Read the model definition and answer for the solid it produces. Units are mm, in the model's axes. A direction names the side the tool comes from. Give positions to 0.01 mm unless a question says otherwise; leave off trailing zeros. Write each loop counter-clockwise with the first axis right and the second up, starting at its lowest first coordinate (ties: lowest second). Pieces come first, ordered by that corner, then holes. Notation, with made-up numbers: M 45.5,-30 L 98.5,-30 A32 cw 98.5,3 Z; hole C 59.25,-16.75 d11. An arc over 180 degrees is marked long. Put each result on its own line as item: value.
from build123d import *

# Parameters (mm, degrees)
SKETCH_1_R               = 18.5
EXTRUDE_1_DEPTH          = 21.5
SKETCH_2_R               = 6
EXTRUDE_2_DEPTH          = 6
SKETCH_3_R               = 3
EXTRUDE_3_DEPTH          = 15
CUT_EXTRUDE_1_DEPTH      = 1
CUT_EXTRUDE_1_DEPTH_BACK = 11.5
SKETCH_5_R               = 1.5
CUT_EXTRUDE_2_DEPTH      = 5
SKETCH_6_R               = 16.4
EXTRUDE_4_DEPTH          = 22
SKETCH_7_R               = 1
EXTRUDE_5_DEPTH          = 6.84
SKETCH_8_R               = 3.75
EXTRUDE_6_DEPTH          = 3.5
SKETCH_9_W               = 0.5
SKETCH_9_H               = 3
EXTRUDE_7_DEPTH          = 6.64


with BuildPart() as part:
    # 草图1 → 凸台-拉伸1 (new body)
    with BuildSketch(Plane.XY):
        Circle(SKETCH_1_R)
    extrude(amount=EXTRUDE_1_DEPTH)

    # 草图2 → 凸台-拉伸2 (add)
    with BuildSketch(Plane(origin=(0, 0, 0), x_dir=(-1, 0, 0), z_dir=(0, 0, -1))):
        with Locations((0, 7)):
            Circle(SKETCH_2_R)
    extrude(amount=EXTRUDE_2_DEPTH)

    # 草图3 → 凸台-拉伸3 (add)
    with BuildSketch(Plane(origin=(0, 0, -6), x_dir=(-1, 0, 0), z_dir=(0, 0, -1))):
        with Locations((0, 7)):
            Circle(SKETCH_3_R)
    extrude(amount=EXTRUDE_3_DEPTH)

    # 草图4 → 切除-拉伸1 (cut, two sides)
    with BuildSketch(Plane(origin=(0, 0, -21), x_dir=(-1, 0, 0), z_dir=(0, 0, -1))) as cut_extrude_1_sk:
        Polygon((-80.661429966, 9.5), (-1.658312395, 9.5), (1.658312395, 9.5), (80.661429966, 9.5), (80.661429966, 167.506235142), (-80.661429966, 167.506235142), align=None)
    extrude(amount=CUT_EXTRUDE_1_DEPTH, mode=Mode.SUBTRACT)
    extrude(cut_extrude_1_sk.sketch, amount=-CUT_EXTRUDE_1_DEPTH_BACK, mode=Mode.SUBTRACT)

    # 草图5 → 切除-拉伸2 (cut)
    with BuildSketch(Plane(origin=(0, 0, 0), x_dir=(-1, 0, 0), z_dir=(0, 0, -1))):
        with Locations((15.5, 0)):
            Circle(SKETCH_5_R)
        with Locations((7.75, -13.423393759)):
            Circle(SKETCH_5_R)
        with Locations((-7.75, -13.423393759)):
            Circle(SKETCH_5_R)
        with Locations((-15.5, 0)):
            Circle(SKETCH_5_R)
        with Locations((-7.75, 13.423393759)):
            Circle(SKETCH_5_R)
        with Locations((7.75, 13.423393759)):
            Circle(SKETCH_5_R)
    extrude(amount=-CUT_EXTRUDE_2_DEPTH, mode=Mode.SUBTRACT)

    # 草图6 → 凸台-拉伸4 (add)
    with BuildSketch(Plane.XY.offset(21.5)):
        Circle(SKETCH_6_R)
    extrude(amount=EXTRUDE_4_DEPTH)

    # 草图7 → 凸台-拉伸5 (add)
    with BuildSketch(Plane.XY.offset(43.5)):
        Circle(SKETCH_7_R)
    extrude(amount=EXTRUDE_5_DEPTH)

    # 草图8 → 凸台-拉伸6 (add)
    with BuildSketch(Plane.XY.offset(43.5)):
        Circle(SKETCH_8_R)
    extrude(amount=EXTRUDE_6_DEPTH)

    # 草图9 → 凸台-拉伸7 (add)
    with BuildSketch(Plane.XY.offset(43.5)):
        with Locations((-12, 0)):
            Rectangle(SKETCH_9_W, SKETCH_9_H)
        with Locations((12, 0)):
            Rectangle(SKETCH_9_W, SKETCH_9_H)
    extrude(amount=EXTRUDE_7_DEPTH)


solid = part.part
(1) Section A-A on x = 0 is taken. Determine the outline of the cut face in (y, z), and give its area (3 significant figures).
Result:
outline: M -18.5,0 L 1,0 L 1,-6 L 4,-6 L 4,-21 L 9.5,-21 L 9.5,-9.5 L 10,-9.5 L 10,-6 L 13,-6 L 13,0 L 18.5,0 L 18.5,21.5 L 16.4,21.5 L 16.4,43.5 L 3.75,43.5 L 3.75,47 L 1,47 L 1,50.34 L -1,50.34 L -1,47 L -3.75,47 L -3.75,43.5 L -16.4,43.5 L -16.4,21.5 L -18.5,21.5 Z
area: 1,710 mm²
(2) Section C-C on z = -2.5 is taken. Determine the outline of the cut face in (x, y).
Result:
outline: C 0,7 d12
(3) Section B-B on y = -6 is taken. Determine the outline of the cut face in (x, z).
Result:
outline: M -17.5,0 L 17.5,0 L 17.5,21.5 L 15.26,21.5 L 15.26,43.5 L -15.26,43.5 L -15.26,21.5 L -17.5,21.5 Z
(4) Given pin 1 Ø6 at (x, z) = (7, 32.5) entering from +Y; pin 2 Ø3.5 at (x, y) = (-16, 0.5) entering from -Z; pin 3 Ø8 at (y, z) = (9, 43) entering from -X, each flat-ended and moving along its own axis, determine where each tip first touches the part or whether it passes through.
Result:
pin 1: stops at y = 15.9
pin 2: stops at z = 0
pin 3: stops at x = -15.62
(5) Straight lines are drawn through the part: line 1 along Y through (x, z) = (7.75, 2.2); line 2 along X through (y, z) = (1, 46.5); line 3 along Z through (x, y) = (5.5, -15.5). For each, find the intervals that lie inside material, in ascending order. Write a range as from..to.
Result:
line 1: y = -16.8..-14.92, -11.92..11.92, 14.92..16.8
line 2: x = -12.25..-11.75, -3.61..3.61, 11.75..12.25
line 3: z = 0..21.5
(6) Which of the six approach directions +Z, -Z, +X, -X, +Y, -Y give full straight-line access (tool end or side, diameter ignored) to faces 1 (the face through (0.78, 12.95, -2.96)), 2 (the face through (-12.25, 0, 47)), 3 (the face through (-2.13, 16.26, 32.35))?
Result:
face 1: -Z
face 2: +Z, -X, +Y, -Y
face 3: +Z
(7) For a pull along Y with two mould halves and no side action, classify faces 4 (the face through (-14, 0, 2)), 5 (the face through (-3.746, 0.165, 45.226)), 6 (the face through (0, 0, 0)), 7 (the face through (8.856, -12.41, 2.465)) as +Y half, -Y half, draft (parallel to the pull), parting line (faces both ways), or undercut.
Result:
face 4: undercut
face 5: parting line
face 6: draft
face 7: undercut
(8) Section D-D on x = 15.5 is taken. Determine the outline of the cut face in (y, z).
Result:
outline: M -10.1,0 L -1.5,0 L -1.5,5 L 1.5,5 L 1.5,0 L 10.1,0 L 10.1,21.5 L 5.36,21.5 L 5.36,43.5 L -5.36,43.5 L -5.36,21.5 L -10.1,21.5 Z
